from build123d import *

# Parameters (mm, degrees)
EXTRUDE_1_DEPTH     = 1.5
SKETCH_2_R          = 1.6
CUT_EXTRUDE_1_DEPTH = 3
SKETCH_3_R          = 1.55
SKETCH_3_R_2        = 3.55
CUT_EXTRUDE_2_DEPTH = 3


with BuildPart() as part:
    # 草图1 → 凸台-拉伸1 (new, symmetric)
    with BuildSketch(Plane.XY):
        with BuildLine():
            Line((-25, 0), (0, 0))
            Line((0, 0), (0, 18))
            ThreePointArc((0, 18), (-12.5, 30.5), (-25, 18))
            Line((-25, 18), (-25, 0))
        make_face()
    extrude(amount=EXTRUDE_1_DEPTH, both=True)

    # 草图2 → 切除-拉伸1 (cut)
    with BuildSketch(Plane.XY.offset(1.5)):
        with Locations((-18, 3.75)):
            Circle(SKETCH_2_R)
        with Locations((-7, 3.75)):
            Circle(SKETCH_2_R)
    extrude(amount=-CUT_EXTRUDE_1_DEPTH, mode=Mode.SUBTRACT)

    # 草图3 → 切除-拉伸2 (cut)
    with BuildSketch(Plane.XY.offset(1.5)):
        with Locations((-4, 18)):
            Circle(SKETCH_3_R)
        with Locations((-21, 18)):
            Circle(SKETCH_3_R)
        with Locations((-12.5, 18)):
            Circle(SKETCH_3_R_2)
    extrude(amount=-CUT_EXTRUDE_2_DEPTH, mode=Mode.SUBTRACT)


solid = part.part
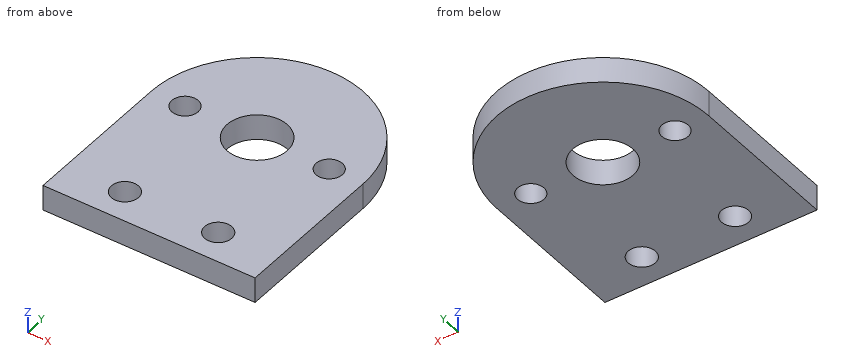
The listing builds one solid part. Answer for the finished solid, in the listing's coordinates (mm). Coordinates: 2 decimals unless noted, no trailing zeros. Loops run counter-clockwise (first coordinate to the right, second up) from the corner with the lowest first, then second, coordinate; pieces in that order, holes last.
1) Find section B-B on z = -0.15. Write down the section's boundary in (x, y), then the cut area to 3 significant figures.
2) Find section D-D on x = -18. Write down the section's boundary in (y, z).
3) Find section A-A on y = 3.75. Write down the section's boundary in (x, z), then the cut area to 3 significant figures.
4) Find section C-C on x = -12.5. Write down the section's boundary in (y, z).
5) Find the intervals of material crossed by L1, parallel to Y at x = -7, z = 0.05; L2, parallel to Y at x = -16.75, z = 0.5; L3, parallel to X at y = 15, z = -0.25, in increasing order.
Values:
1. outline: (-25, 0) - (0, 0) - (0, 18) arc R12.5 ccw to (-25, 18) - close; hole circle Ø3.1 at (-21, 18); hole circle Ø3.2 at (-18, 3.75); hole circle Ø7.1 at (-12.5, 18); hole circle Ø3.2 at (-7, 3.75); hole circle Ø3.1 at (-4, 18)
1. area: 625 mm2
2. outline: (0, -1.5) - (2.15, -1.5) - (2.15, 1.5) - (0, 1.5) - close; (5.35, -1.5) - (29.22, -1.5) - (29.22, 1.5) - (5.35, 1.5) - close
3. outline: (-25, -1.5) - (-19.6, -1.5) - (-19.6, 1.5) - (-25, 1.5) - close; (-16.4, -1.5) - (-8.6, -1.5) - (-8.6, 1.5) - (-16.4, 1.5) - close; (-5.4, -1.5) - (0, -1.5) - (0, 1.5) - (-5.4, 1.5) - close
3. area: 55.8 mm2
4. outline: (0, -1.5) - (14.45, -1.5) - (14.45, 1.5) - (0, 1.5) - close; (21.55, -1.5) - (30.5, -1.5) - (30.5, 1.5) - (21.55, 1.5) - close
5. L1: y = 0 to 2.15, 5.35 to 29.22
5. L2: y = 0 to 2.75, 4.75 to 29.76
5. L3: x = -25 to -14.4, -10.6 to 0
